Design review of the part built by this model. Coordinates are the model's own, in mm. A direction names the side the tool comes from. Round coordinates to 2 decimals unless told otherwise and drop trailing zeros. Loops run counter-clockwise (first coordinate to the right, second up) from the corner with the lowest first, then second, coordinate; pieces in that order, holes last. Notation, with made-up numbers: M -36,43 L 6,43 A22 ccw 6,78 Z; hole C 56.25,-5.5 d8. An arc over 180 degrees is marked long. One line per item, written item: value. Start each with the question number.
Item 1: For faces 4 (the cylindrical face through (-80.57, 154.89, 2.96)), 5 (the cylindrical face through (-90.955, 140.265, 2.958)), list the 3-axis set-ups (+Z, -Z, +X, -X, +Y, -Y) from which the entire face can be reached by the end or side of a thin tool; tool diameter is ignored.
Item 2: For line 1 along X through (y, z) = (148.5, 4.4); line 2 along Y through (x, z) = (-81, 4.25); line 3 along X through (y, z) = (146.5, 3.05), list the stretches that pass through material, from the lowest coordinate up.
Item 3: We need section B-B (y = 101). Write out the cut boundary in (x, z), then the cut area to 3 significant figures.
Item 4: Mouldability with a two-part tool opening along X and no side actions: class faces 1 (the flat face through (-80.139, 166.984, 2.958)), 2 (the cylindrical face through (-6.238, 21.355, 2.958)), 3 (the flat face through (-50, 88, 0)) as released by +X, released by -X, zero draft, split by the parting line, or undercut.
Item 5: We need section A-A (z = 4.2). State how many separate pieces and enclosed holes the cut face has, then the cut area to 3 significant figures.
Item 6: Clearance check with flat-ended pins moving along their axes: pin 1 (5.5 mm diameter, centred on x = -77.31, y = 146.5, fed in from +Z); pin 2 (1 mm diameter, centred on x = -76, z = 5, fed in from -Y); pin 3 (1.5 mm diameter, centred on x = -21, z = 2, fed in from +Y); pin 4 (1.5 mm diameter, centred on y = 94.5, z = 1.5, fed in from -X). State where each tip first meets the part, or that it passes through.
from build123d import *

# Parameters (mm, degrees)
CROQUIS1_R              = 3.4
CROQUIS1_R_2            = 3
CROQUIS1_R_3            = 1.5
CROQUIS1_R_4            = 1.500001004
SALIENTE_EXTRUIR1_DEPTH = 6


with BuildPart() as part:
    # Croquis1 → Saliente-Extruir1 (new body)
    with BuildSketch(Plane.XY):
        with BuildLine():
            Line((-29.303608517, 45.473325839), (-58.336924517, 119.389926839))
            ThreePointArc((-58.336924517, 119.389926839), (-61.793103757, 132.204361213), (-62.347490923, 145.46511376))
            ThreePointArc((-62.347490923, 145.46511376), (-63.047561651, 151.140362617), (-65.820602243, 156.141241988))
            Line((-65.820602243, 156.141241988), (-79.226205243, 172.119032988))
            ThreePointArc((-79.226205243, 172.119032988), (-88.279569401, 174.423233147), (-93.344634593, 166.573528977))
            Line((-93.344634593, 166.573528977), (-92.292655243, 145.743421988))
            ThreePointArc((-92.292655243, 145.743421988), (-90.920958081, 140.192116496), (-87.571476882, 135.557516032))
            ThreePointArc((-87.571476882, 135.557516032), (-78.952780907, 125.464301499), (-72.763926988, 113.723220326))
            Line((-72.763926988, 113.723220326), (-42.706743988, 37.199930326))
            ThreePointArc((-42.706743988, 37.199930326), (-42.359256153, 36.438795137), (-41.931739661, 35.719556497))
            Line((-41.931739661, 35.719556497), (-17.999999661, 4.97e-07))
            Line((-17.999999661, 4.97e-07), (-2.999999661, 4.97e-07))
            ThreePointArc((-2.999999661, 4.97e-07), (-0.878679318, 0.878680154), (3.39e-07, 3.000000497))
            Line((3.39e-07, 3.000000497), (3.39e-07, 14.250000497))
            Line((3.39e-07, 14.250000497), (-4.079708661, 19.244683497))
            ThreePointArc((-4.079708661, 19.244683497), (-6.27155818, 21.381766981), (-8.886999737, 22.972614423))
            ThreePointArc((-8.886999737, 22.972614423), (-12.726828858, 25.305121653), (-15.949120882, 28.435890212))
            Line((-15.949120882, 28.435890212), (-27.725819882, 42.785152212))
            ThreePointArc((-27.725819882, 42.785152212), (-28.620096035, 44.067386525), (-29.303608517, 45.473325839))
        make_face()
        with Locations((-77.311748512, 146.499999762)):
            Circle(CROQUIS1_R, mode=Mode.SUBTRACT)
        with Locations((-15.25, 15.25)):
            Circle(CROQUIS1_R_2, mode=Mode.SUBTRACT)
        with Locations((-25.371621, 27.641642)):
            Circle(CROQUIS1_R_3, mode=Mode.SUBTRACT)
        with Locations((-35.49324282, 40.033285892)):
            Circle(CROQUIS1_R_4, mode=Mode.SUBTRACT)
        with BuildLine():
            Line((-71.99439, 154.818095), (-72.793676, 152.984753))
            ThreePointArc((-72.793676, 152.984753), (-74.833795849, 152.18374175), (-75.635356, 154.223646))
            Line((-75.635356, 154.223646), (-74.836069921, 156.056987462))
            ThreePointArc((-74.836069921, 156.056987462), (-72.795783729, 156.858381191), (-71.99439, 154.818095))
        make_face(mode=Mode.SUBTRACT)
        with BuildLine():
            Line((-86.868735462, 148.975678079), (-85.035394, 148.176392))
            ThreePointArc((-85.035394, 148.176392), (-82.9951075, 148.9777855), (-83.796501, 151.018072))
            Line((-83.796501, 151.018072), (-85.629843, 151.817358))
            ThreePointArc((-85.629843, 151.817358), (-87.669747153, 151.015797712), (-86.868735462, 148.975678079))
        make_face(mode=Mode.SUBTRACT)
        with BuildLine():
            Line((-67.754760538, 144.024321921), (-69.588102, 144.823608))
            ThreePointArc((-69.588102, 144.823608), (-71.62800625, 144.022047849), (-70.826995, 141.981928))
            Line((-70.826995, 141.981928), (-68.993653, 141.182642))
            ThreePointArc((-68.993653, 141.182642), (-66.953366809, 141.98403573), (-67.754760538, 144.024321921))
        make_face(mode=Mode.SUBTRACT)
        with BuildLine():
            Line((-82.89780493, 154.919280048), (-86.61137993, 156.538295048))
            ThreePointArc((-86.61137993, 156.538295048), (-88.302670061, 157.929718336), (-89.007717, 160.003225))
            Line((-89.007717, 160.003225), (-89.349725675, 166.775282995))
            ThreePointArc((-89.349725675, 166.775282995), (-86.817213433, 170.700127324), (-82.290539057, 169.548068144))
            Line((-82.290539057, 169.548068144), (-77.926769806, 164.347120835))
            ThreePointArc((-77.926769806, 164.347120835), (-77.036994499, 162.350360642), (-77.32981093, 160.184025048))
            Line((-77.32981093, 160.184025048), (-78.94886318, 156.470364412))
            ThreePointArc((-78.94886318, 156.470364412), (-80.602093919, 154.876969498), (-82.89780493, 154.919280048))
        make_face(mode=Mode.SUBTRACT)
        with BuildLine():
            Line((-82.629106, 138.181905), (-81.82982, 140.015247))
            ThreePointArc((-81.82982, 140.015247), (-79.7895335, 140.8166405), (-78.98814, 138.776354))
            Line((-78.98814, 138.776354), (-79.787426079, 136.943012538))
            ThreePointArc((-79.787426079, 136.943012538), (-81.827545712, 136.142000847), (-82.629106, 138.181905))
        make_face(mode=Mode.SUBTRACT)
    extrude(amount=SALIENTE_EXTRUIR1_DEPTH)


solid = part.part
A:
1. face 4: +Z, -Z
1. face 5: +Z, -Z, -X, -Y
2. line 1: -92.43 to -85.78, -83.32 to -80.06, -74.56 to -62.45
2. line 2: 128.3 to 136.03, 140.83 to 154.75, 168.01 to 173.69
2. line 3: -92.33 to -80.71, -73.91 to -62.31
3. outline: M -67.77,0 L -51.11,0 L -51.11,6 L -67.77,6 Z
3. area: 99.9 mm2
4. face 1: undercut
4. face 2: released by +X
4. face 3: zero draft
5. separate pieces: 1
5. enclosed holes: 9
5. area: 3,220 mm2
6. pin 1: through
6. pin 2: y = 119.7
6. pin 3: y = 35.5
6. pin 4: x = -65.51
